Check sheet for the drawn part. Datum: minimum x, y, z corner. Units: mm. Round coordinates to 2 decimals unless told otherwise and drop trailing zeros. Order: outer loops, then holes, each group sorted by start corner. A loop starts at its lowest first (then second) coordinate and runs counter-clockwise, first axis right, second up. Notation, with made-up numbers: (21.5, 11) -> (47.5, 11) arc R11 cw to (47.5, 20) -> close; hole circle Ø10 at (4.25, -23). An arc over 180 degrees is marked (long way). Answer as a JSON object with one key per item and string values. Group by question number.
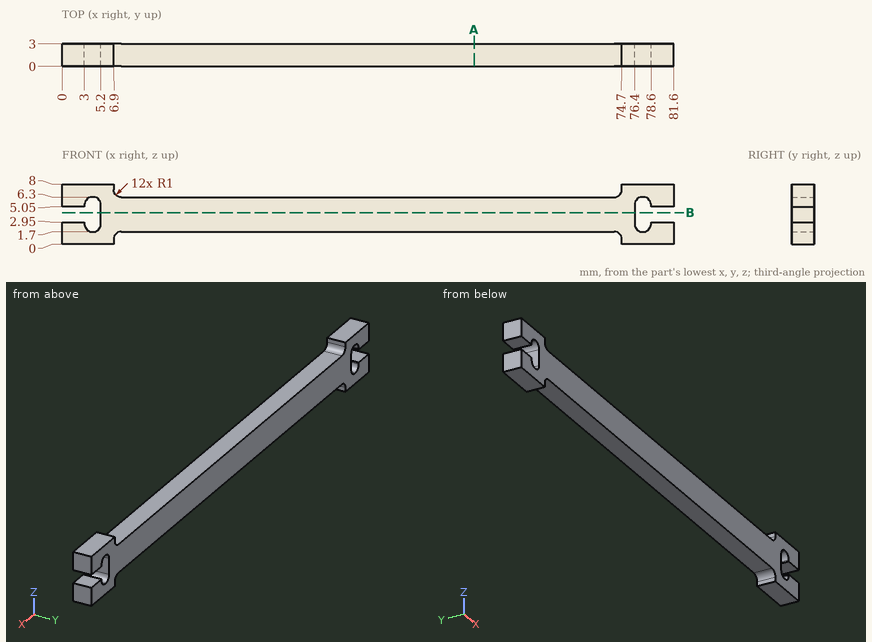
Item 1: Thickness scan on L1, parallel to X at y = 1.2, z = 2.75; L2, parallel to X at y = 1.25, z = 0.5; L3, parallel to X at y = 1.7, z = 5.75. Record the ranges inside material, lowest first.
Item 2: Sectioned sample at A-A, the plane x = 55. Enter the section's corners in (y, z).
Item 3: Depth check by flat-ended pin: pin 1 Ø1.3 at (y, z) = (2, 3.5) entering from +X; pin 2 Ø1 at (x, y) = (29.5, 1.5) entering from -Z; pin 3 Ø0.8 at (y, z) = (1, 3.5) entering from -X. Enter the tip coordinate at first touch or a pass-through.
Item 4: Sectioned sample at B-B, the plane z = 4.25. Enter the section's corners in (x, y), then the cut area to 3 significant figures.
Result:
{
 "1": {"L1": "x = 0 to 3, 5.2 to 76.4, 78.6 to 81.6", "L2": "x = 0 to 6.9, 74.7 to 81.6", "L3": "x = 0 to 3.11, 5.09 to 76.51, 78.49 to 81.6"},
 "2": {"outline": "(0, 1.7) -> (3, 1.7) -> (3, 6.3) -> (0, 6.3) -> close"},
 "3": {"pin 1": "stops at x = 81.6", "pin 2": "stops at z = 1.7", "pin 3": "stops at x = 5.2"},
 "4": {"outline": "(5.2, 0) -> (76.4, 0) -> (76.4, 3) -> (5.2, 3) -> close", "area": "214 mm2"}
}
